For this review, take the finished solid that the model builds, in its own axes (mm). A direction names the side the tool comes from. Give positions to 0.01 mm unless a question says otherwise; leave off trailing zeros. Loops run counter-clockwise (first coordinate to the right, second up) from the corner with the lowest first, then second, coordinate; pieces in that order, holes last. Notation, with made-up numbers: (-23, 40.25) - (-2, 40.25) arc R23 cw to (-2, 52.25) - close; hole circle Ø7 at (52.25, 19). An arc over 180 degrees is marked (long way). Use CSV: the item, a comma, the result in double quotes. Start each with the question number.
1. Mouldability with a two-part tool opening along Z and no side actions: class faces 1 (the flat face through (39, 5, -33)), 2 (the flat face through (53, 2, -2.75)), 3 (the cylindrical face through (12.142, 2.465, -45.227)) as pulls with the +Z half, pulls with the -Z half, needs draft (parallel to the pull), parting line crosses it, or undercut.
2. Wall thickness on line 1 (Z direction, x = 27, y = 3.2); line 2 (Z direction, x = 29.5, y = 4.7); line 3 (X direction, y = 1.4, z = -32.5): over which ranges is each line inside the solid? List them lowest first.
3. Take a section at B-B on x = 34. State how many separate pieces and enclosed holes the cut face has, plus the area to 3 significant figures.
4. For pin 1 (3.5 mm diameter, centred on x = 32.5, z = -22.5, fed in from -Y), flat-tipped, find the tip position at first contact; note if it passes through.
5. Take a section at C-C on z = -31. Give the boundary of the cut face in (x, y), plus the area to 3 significant figures.
6. For faces 4 (the cylindrical face through (19.75, 2.46, -52.44)), 5 (the cylindrical face through (47.005, 4.014, -32.742)), 6 (the flat face through (0, 2, -32)), list the 3-axis set-ups (+Z, -Z, +X, -X, +Y, -Y) from which the entire face can be reached by the end or side of a thin tool; tool diameter is ignored.
7. Take a section at A-A on z = -12.5. Give the boundary of the cut face in (x, y).
```python
from build123d import *

# Parameters (mm, degrees)
SKETCH1_W           = 65
SKETCH1_H           = 65
SKETCH1_R           = 2.75
SKETCH1_R_2         = 3.75
BOSS_EXTRUDE1_DEPTH = 5
SKETCH2_R           = 5.5
CUT_EXTRUDE1_DEPTH  = 2


with BuildPart() as part:
    # Sketch1 → Boss-Extrude1 (new body)
    with BuildSketch(Plane(origin=(0, 0, 0), x_dir=(1, 0, 0), z_dir=(0, 1, 0))):
        with Locations((32.5, 32.5)):
            Rectangle(SKETCH1_W, SKETCH1_H)
        with Locations((32.5, 32.5)):
            Circle(SKETCH1_R, mode=Mode.SUBTRACT)
        with Locations((22.5, 32.5)):
            Circle(SKETCH1_R, mode=Mode.SUBTRACT)
        with Locations((12.5, 32.5)):
            Circle(SKETCH1_R, mode=Mode.SUBTRACT)
        with Locations((32.5, 42.5)):
            Circle(SKETCH1_R, mode=Mode.SUBTRACT)
        with Locations((12.5, 42.5)):
            Circle(SKETCH1_R, mode=Mode.SUBTRACT)
        with Locations((12.5, 52.5)):
            Circle(SKETCH1_R, mode=Mode.SUBTRACT)
        with Locations((42.5, 32.5)):
            Circle(SKETCH1_R, mode=Mode.SUBTRACT)
        with Locations((52.5, 32.5)):
            Circle(SKETCH1_R_2, mode=Mode.SUBTRACT)
        with Locations((52.5, 42.5)):
            Circle(SKETCH1_R, mode=Mode.SUBTRACT)
        with Locations((52.5, 22.5)):
            Circle(SKETCH1_R, mode=Mode.SUBTRACT)
        with Locations((32.5, 22.5)):
            Circle(SKETCH1_R, mode=Mode.SUBTRACT)
        with Locations((12.5, 22.5)):
            Circle(SKETCH1_R, mode=Mode.SUBTRACT)
        with Locations((12.5, 12.5)):
            Circle(SKETCH1_R, mode=Mode.SUBTRACT)
        with Locations((52.5, 52.5)):
            Circle(SKETCH1_R, mode=Mode.SUBTRACT)
        with Locations((52.5, 12.5)):
            Circle(SKETCH1_R, mode=Mode.SUBTRACT)
        with BuildLine():
            Line((22.5, 55.25), (42.5, 55.25))
            ThreePointArc((42.5, 55.25), (45.25, 52.5), (42.5, 49.75))
            Line((42.5, 49.75), (22.5, 49.75))
            ThreePointArc((22.5, 49.75), (19.75, 52.5), (22.5, 55.25))
        make_face(mode=Mode.SUBTRACT)
        with BuildLine():
            Line((29.25, 62.25), (35.75, 62.25))
            ThreePointArc((35.75, 62.25), (37.5, 60.5), (35.75, 58.75))
            Line((35.75, 58.75), (29.25, 58.75))
            ThreePointArc((29.25, 58.75), (27.5, 60.5), (29.25, 62.25))
        make_face(mode=Mode.SUBTRACT)
        with BuildLine():
            Line((9.25, 62.25), (15.75, 62.25))
            ThreePointArc((15.75, 62.25), (17.5, 60.5), (15.75, 58.75))
            Line((15.75, 58.75), (9.25, 58.75))
            ThreePointArc((9.25, 58.75), (7.5, 60.5), (9.25, 62.25))
        make_face(mode=Mode.SUBTRACT)
        with BuildLine():
            Line((55.75, 62.25), (49.25, 62.25))
            ThreePointArc((49.25, 62.25), (47.5, 60.5), (49.25, 58.75))
            Line((49.25, 58.75), (55.75, 58.75))
            ThreePointArc((55.75, 58.75), (57.5, 60.5), (55.75, 62.25))
        make_face(mode=Mode.SUBTRACT)
        with BuildLine():
            Line((22.5, 9.75), (42.5, 9.75))
            ThreePointArc((42.5, 9.75), (45.25, 12.5), (42.5, 15.25))
            Line((42.5, 15.25), (22.5, 15.25))
            ThreePointArc((22.5, 15.25), (19.75, 12.5), (22.5, 9.75))
        make_face(mode=Mode.SUBTRACT)
        with BuildLine():
            Line((55.75, 2.75), (49.25, 2.75))
            ThreePointArc((49.25, 2.75), (47.5, 4.5), (49.25, 6.25))
            Line((49.25, 6.25), (55.75, 6.25))
            ThreePointArc((55.75, 6.25), (57.5, 4.5), (55.75, 2.75))
        make_face(mode=Mode.SUBTRACT)
        with BuildLine():
            Line((9.25, 2.75), (15.75, 2.75))
            ThreePointArc((15.75, 2.75), (17.5, 4.5), (15.75, 6.25))
            Line((15.75, 6.25), (9.25, 6.25))
            ThreePointArc((9.25, 6.25), (7.5, 4.5), (9.25, 2.75))
        make_face(mode=Mode.SUBTRACT)
        with BuildLine():
            Line((29.25, 2.75), (35.75, 2.75))
            ThreePointArc((35.75, 2.75), (37.5, 4.5), (35.75, 6.25))
            Line((35.75, 6.25), (29.25, 6.25))
            ThreePointArc((29.25, 6.25), (27.5, 4.5), (29.25, 2.75))
        make_face(mode=Mode.SUBTRACT)
    extrude(amount=BOSS_EXTRUDE1_DEPTH)

    # Sketch2 → Cut-Extrude1 (cut)
    with BuildSketch(Plane(origin=(0, 5, 0), x_dir=(1, 0, 0), z_dir=(0, 1, 0))):
        with Locations((12.5, 52.5)):
            Circle(SKETCH2_R)
        with Locations((52.5, 32.5)):
            Circle(SKETCH2_R)
        with Locations((12.5, 12.5)):
            Circle(SKETCH2_R)
    extrude(amount=-CUT_EXTRUDE1_DEPTH, mode=Mode.SUBTRACT)


solid = part.part
```
Check result:
1,face 1,"needs draft"
1,face 2,"undercut"
1,face 3,"undercut"
2,line 1,"z = -65 to -55.25, -49.75 to -15.25, -9.75 to 0"
2,line 2,"z = -65 to -62.25, -58.75 to -55.25, -49.75 to -15.25, -9.75 to -6.25, -2.75 to 0"
2,line 3,"x = 0 to 9.75, 15.25 to 19.75, 25.25 to 29.75, 35.25 to 39.75, 45.25 to 48.75, 56.25 to 65"
3,separate pieces,"8"
3,enclosed holes,"0"
3,area,"166 mm²"
4,pin 1,"passes through"
5,outline,"(0, 0) - (10.2, 0) - (10.2, 5) - (0, 5) - close; (14.8, 0) - (20.2, 0) - (20.2, 5) - (14.8, 5) - close; (24.8, 0) - (30.2, 0) - (30.2, 5) - (24.8, 5) - close; (34.8, 0) - (40.2, 0) - (40.2, 5) - (34.8, 5) - close; (44.8, 0) - (49.06, 0) - (49.06, 3) - (47.21, 3) - (47.21, 5) - (44.8, 5) - close; (55.94, 0) - (65, 0) - (65, 5) - (57.79, 5) - (57.79, 3) - (55.94, 3) - close"
5,area,"191 mm²"
6,face 4,"+Y, -Y"
6,face 5,"+Y"
6,face 6,"+Z, -Z, -X, +Y, -Y"
7,outline,"(0, 0) - (9.75, 0) - (9.75, 3) - (7, 3) - (7, 5) - (0, 5) - close; (15.25, 0) - (19.75, 0) - (19.75, 5) - (18, 5) - (18, 3) - (15.25, 3) - close; (45.25, 0) - (49.75, 0) - (49.75, 5) - (45.25, 5) - close; (55.25, 0) - (65, 0) - (65, 5) - (55.25, 5) - close"
